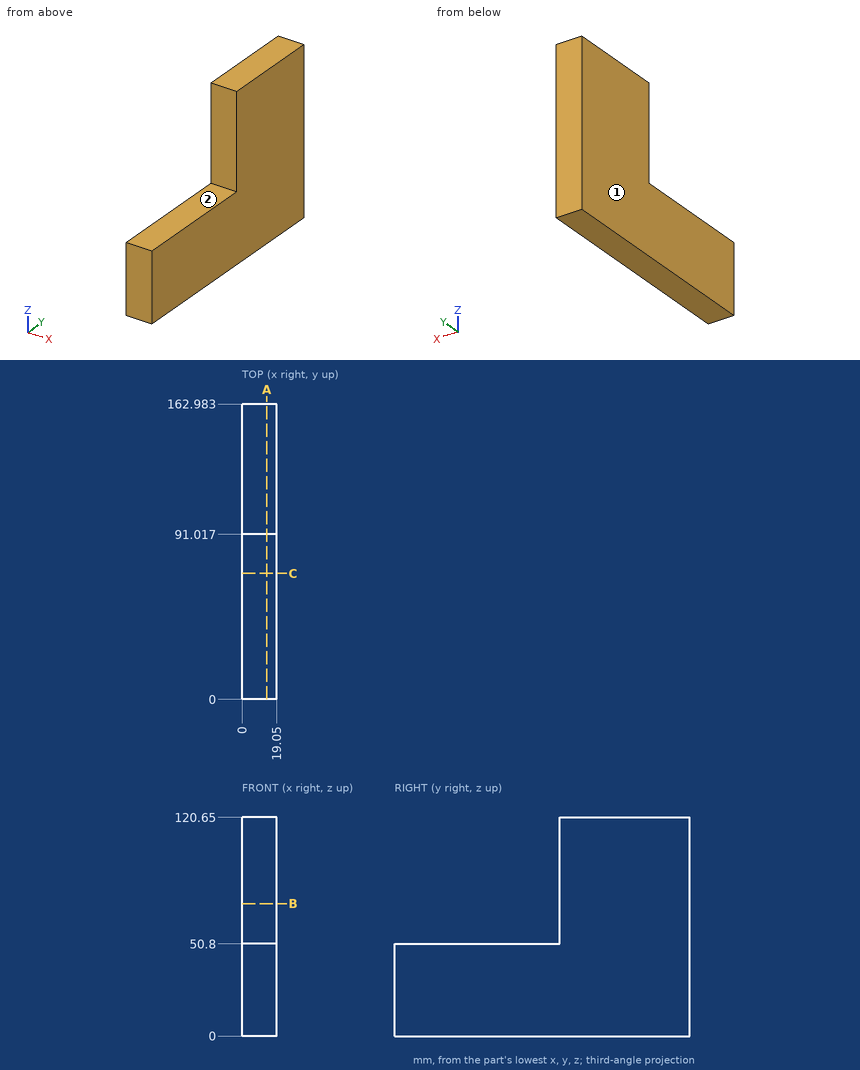
Here's the drawing with two shaded views (mm, measured from the low corner). I have some questions. A direction names the side the tool comes from. Coordinates: 2 decimals unless noted, no trailing zeros. Order: outer loops, then holes, each group sorted by start corner. A loop starts at its lowest first (then second) coordinate and runs counter-clockwise, first axis right, second up. Notation, with made-up numbers: (-29.5, 32.25) - (-1.5, 32.25) arc R8 cw to (-1.5, 42.25) - close; hole circle Ø3 at (45, -28). An arc over 180 degrees is marked (long way). Use CSV: the item, a comma, the result in double quotes. Start each with the question number.
1. I'm going to push flat-ended pins straight in: pin 1 (6 mm diameter, centred on x = 12, y = 96.5, fed in from -Z); pin 2 (9.5 mm diameter, centred on x = 9, z = 75, fed in from -Y); pin 3 (1 mm diameter, centred on x = 12.5, y = 71.5, fed in from +Z). Where does each tip first touch, or does it pass through?
2. Suppose I cut it at B-B on z = 73. List the corners of the cut face in (x, y) for me.
3. For the marked faces 1 and 2, which set-ups out of +Z, -Z, +X, -X, +Y, -Y let a thin tool reach every point of the face, with its end or its side?
4. Suppose I cut it at A-A on x = 13.75. List the corners of the cut face in (y, z) for me, then the cut area to 3 significant figures.
5. Suppose I cut it at C-C on y = 69.5. List the corners of the cut face in (x, z) for me.
6. Please list where these lines run through material, in increasing order: line 1 (Z direction, x = 8, y = 30.5); line 2 (Y direction, x = 14.25, z = 106.5). Write a range as from..to.
Output:
1,pin 1,"stops at z = 0"
1,pin 2,"stops at y = 91.02"
1,pin 3,"stops at z = 50.8"
2,outline,"(0, 91.02) - (19.05, 91.02) - (19.05, 162.98) - (0, 162.98) - close"
3,face 1,"+Z, -Z, -X, +Y, -Y"
3,face 2,"+Z, +X, -X, -Y"
4,outline,"(0, 0) - (162.98, 0) - (162.98, 120.65) - (91.02, 120.65) - (91.02, 50.8) - (0, 50.8) - close"
4,area,"13,300 mm2"
5,outline,"(0, 0) - (19.05, 0) - (19.05, 50.8) - (0, 50.8) - close"
6,line 1,"z = 0..50.8"
6,line 2,"y = 91.02..162.98"
